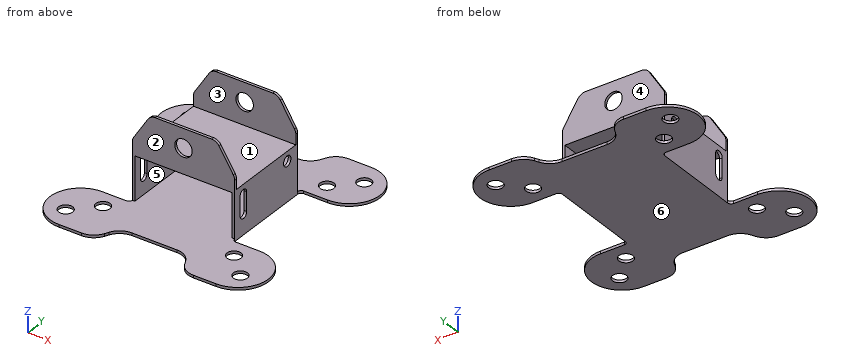
from build123d import *

# Parameters (mm, degrees)
SKETCH1_R           = 4.022928706
BOSS_EXTRUDE1_DEPTH = 1.5
SKETCH3_W           = 1.5
SKETCH3_H           = 50.876500294
BOSS_EXTRUDE2_DEPTH = 25
SKETCH4_W           = 58.54657641
SKETCH4_H           = 50.876500294
BOSS_EXTRUDE3_DEPTH = 1.5
SKETCH5_R           = 5
BOSS_EXTRUDE4_DEPTH = 1.5
SKETCH8_R           = 2.960999365
CUT_EXTRUDE1_DEPTH  = 92.835038059
FILLET1_R           = 5


with BuildPart() as part:
    # Sketch1 → Boss-Extrude1 (new body)
    with BuildSketch(Plane.XY):
        with BuildLine():
            Line((-31.273288205, 27.438250147), (-45, 27.438250147))
            ThreePointArc((-45, 27.438250147), (-62.561749853, 45), (-45, 62.561749853))
            Line((-45, 62.561749853), (-31.990503674, 62.561749853))
            ThreePointArc((-31.990503674, 62.561749853), (-26.633250489, 61.005673012), (-22.943256827, 56.821717516))
            Line((-22.943256827, 56.821717516), (-21.912531254, 54.632680079))
            ThreePointArc((-21.912531254, 54.632680079), (-18.222537592, 50.448724583), (-12.865284407, 48.892647742))
            Line((-12.865284407, 48.892647742), (12.865284407, 48.892647742))
            ThreePointArc((12.865284407, 48.892647742), (18.222537592, 50.448724583), (21.912531254, 54.632680079))
            Line((21.912531254, 54.632680079), (22.943256827, 56.821717516))
            ThreePointArc((22.943256827, 56.821717516), (26.633250489, 61.005673012), (31.990503674, 62.561749853))
            Line((31.990503674, 62.561749853), (45, 62.561749853))
            ThreePointArc((45, 62.561749853), (62.561749853, 45), (45, 27.438250147))
            Line((45, 27.438250147), (31.273288205, 27.438250147))
            ThreePointArc((31.273288205, 27.438250147), (29.859074643, 26.852463709), (29.273288205, 25.438250147))
            Line((29.273288205, 25.438250147), (29.273288205, -25.438250147))
            ThreePointArc((29.273288205, -25.438250147), (29.859074643, -26.852463709), (31.273288205, -27.438250147))
            Line((31.273288205, -27.438250147), (45, -27.438250147))
            ThreePointArc((45, -27.438250147), (62.561749853, -45), (45, -62.561749853))
            Line((45, -62.561749853), (31.990503674, -62.561749853))
            ThreePointArc((31.990503674, -62.561749853), (26.633250489, -61.005673012), (22.943256827, -56.821717516))
            Line((22.943256827, -56.821717516), (21.912531254, -54.632680079))
            ThreePointArc((21.912531254, -54.632680079), (18.222537592, -50.448724583), (12.865284407, -48.892647742))
            Line((12.865284407, -48.892647742), (-12.865284407, -48.892647742))
            ThreePointArc((-12.865284407, -48.892647742), (-18.222537592, -50.448724583), (-21.912531254, -54.632680079))
            Line((-21.912531254, -54.632680079), (-22.943256827, -56.821717516))
            ThreePointArc((-22.943256827, -56.821717516), (-26.633250489, -61.005673012), (-31.990503674, -62.561749853))
            Line((-31.990503674, -62.561749853), (-45, -62.561749853))
            ThreePointArc((-45, -62.561749853), (-62.561749853, -45), (-45, -27.438250147))
            Line((-45, -27.438250147), (-31.273288205, -27.438250147))
            ThreePointArc((-31.273288205, -27.438250147), (-29.859074643, -26.852463709), (-29.273288205, -25.438250147))
            Line((-29.273288205, -25.438250147), (-29.273288205, 25.438250147))
            ThreePointArc((-29.273288205, 25.438250147), (-29.859074643, 26.852463709), (-31.273288205, 27.438250147))
        make_face()
        with Locations((-50, 50)):
            Circle(SKETCH1_R, mode=Mode.SUBTRACT)
        with Locations((50, 50)):
            Circle(SKETCH1_R, mode=Mode.SUBTRACT)
        with Locations((-37.5, 37.5)):
            Circle(SKETCH1_R, mode=Mode.SUBTRACT)
        with Locations((37.5, 37.5)):
            Circle(SKETCH1_R, mode=Mode.SUBTRACT)
        with Locations((50, -50)):
            Circle(SKETCH1_R, mode=Mode.SUBTRACT)
        with Locations((37.5, -37.5)):
            Circle(SKETCH1_R, mode=Mode.SUBTRACT)
        with Locations((-37.5, -37.5)):
            Circle(SKETCH1_R, mode=Mode.SUBTRACT)
        with Locations((-50, -50)):
            Circle(SKETCH1_R, mode=Mode.SUBTRACT)
    extrude(amount=BOSS_EXTRUDE1_DEPTH)

    # Sketch3 → Boss-Extrude2 (add)
    with BuildSketch(Plane.XY.offset(1.5)):
        with Locations((-28.523288205, 0)):
            Rectangle(SKETCH3_W, SKETCH3_H)
        with Locations((28.523288205, 0)):
            Rectangle(SKETCH3_W, SKETCH3_H)
    extrude(amount=BOSS_EXTRUDE2_DEPTH)

    # Sketch4 → Boss-Extrude3 (add)
    with BuildSketch(Plane.XY.offset(26.5)):
        Rectangle(SKETCH4_W, SKETCH4_H)
    extrude(amount=BOSS_EXTRUDE3_DEPTH)

    # Sketch5 → Boss-Extrude4 (add)
    with BuildSketch(Plane(origin=(0, 25.438250147, 0), x_dir=(1, 0, 0), z_dir=(0, 1, 0))):
        Polygon((-29.273288205, -28), (-29.273288205, -35.308019153), (-18.871561113, -51.78577911), (18.871561113, -51.78577911), (29.273288205, -35.308019153), (29.273288205, -28), align=None)
        with Locations((0, -40.861297371)):
            Circle(SKETCH5_R, mode=Mode.SUBTRACT)
    boss_extrude4 = extrude(amount=-BOSS_EXTRUDE4_DEPTH)

    # Mirror1: Boss-Extrude4 across plane
    add(boss_extrude4.mirror(Plane.ZX))

    # Sketch8 → Cut-Extrude1 (cut, through all)
    with BuildSketch(Plane.ZY.offset(29.273288205)):
        with Locations((22.546846222, 17.00872447)):
            Circle(SKETCH8_R)
        with BuildLine():
            Line((11.727810079, -15.733095436), (22.546846222, -15.733095436))
            ThreePointArc((22.546846222, -15.733095436), (25.204153345, -18.390402559), (22.546846222, -21.047709682))
            Line((22.546846222, -21.047709682), (11.727810079, -21.047709682))
            ThreePointArc((11.727810079, -21.047709682), (9.070502956, -18.390402559), (11.727810079, -15.733095436))
        make_face()
    extrude(amount=-CUT_EXTRUDE1_DEPTH, mode=Mode.SUBTRACT)

    # Fillet1
    fillet1_edges = [part.edges().sort_by_distance(p)[0] for p in [
        (29.273288205, 24.688250147, 35.308019153),
        (18.871561113, 24.688250147, 51.78577911),
        (-18.871561113, 24.688250147, 51.78577911),
        (-29.273288205, 24.688250147, 35.308019153),
        (-29.273288205, -24.688250147, 35.308019153),
        (-18.871561113, -24.688250147, 51.78577911),
        (18.871561113, -24.688250147, 51.78577911),
        (29.273288205, -24.688250147, 35.308019153),
    ]]
    fillet(fillet1_edges, radius=FILLET1_R)


solid = part.part
Geometry: final body of the model. Coordinates: model frame, mm. Face numbers are marked on the shaded views. A direction names the side the tool comes from. Give positions to 0.01 mm unless a question says otherwise; leave off trailing zeros. Write each loop counter-clockwise with the first axis right and the second up, starting at its lowest first coordinate (ties: lowest second). Pieces come first, ordered by that corner, then holes. Notation, with made-up numbers: (74, 67) - (107, 67) arc R22 cw to (107, 73) - close; hole circle Ø4 at (8.25, 46.5). An arc over 180 degrees is marked (long way). Return JSON: item names as keys, results as strings. Group by question number.
1) Line query: line 1 (X direction, y = -20.5, z = 25.5); line 2 (Y direction, x = 16.5, z = 48.5); line 3 (Z direction, x = 0, y = -24.7). Output: solid intervals per line, ascending.
2) Section A-A on x = 0. Return the cut outline in (y, z).
3) Set-up query: the marked faces 5 and 6. Return all of +Z, -Z, +X, -X, +Y, -Y with unobstructed straight access to the full face (end or side cutting, diameter ignored); none if empty.
4) Mould query, pull axis Y, two halves, no side actions, for the marked faces 1, 2, 3 and 4. Classes: released by +Y, released by -Y, zero draft, split by the parting line, or undercut.
5) Section C-C on x = -43. Return the cut outline in (y, z), plus the area to 3 significant figures.
6) Section D-D on y = -0.5. Return the cut outline in (x, z), plus the area to 3 significant figures.
7) First-contact query: P1, Ø12, axis at y = 19, z = 18, coming from the -X side; P2, Ø3, axis at x = 32, y = -8.5, coming from the +Z side; P3, Ø5, axis at y = -8.5, z = 8.5, coming from the +X side; P4, Ø2, axis at x = 28, y = -32, coming from the +Z side. Flat tips, straight axial feed; report the tip coordinate or a pass-through.
8) Section B-B on z = 3. Return the cut outline in (x, y).
Filled in:
{
 "1": {"line 1": "x = -29.27 to -27.77, 27.77 to 29.27", "line 2": "y = -25.44 to -23.94, 23.94 to 25.44", "line 3": "z = 0 to 1.5, 26.5 to 35.86, 45.86 to 51.79"},
 "2": {"outline": "(-48.89, 0) - (48.89, 0) - (48.89, 1.5) - (-48.89, 1.5) - close; (-25.44, 26.5) - (25.44, 26.5) - (25.44, 35.86) - (23.94, 35.86) - (23.94, 28) - (-23.94, 28) - (-23.94, 35.86) - (-25.44, 35.86) - close; (-25.44, 45.86) - (-23.94, 45.86) - (-23.94, 51.79) - (-25.44, 51.79) - close; (23.94, 45.86) - (25.44, 45.86) - (25.44, 51.79) - (23.94, 51.79) - close"},
 "3": {"face 5": "+Y, -Y", "face 6": "-Z, +X, -X, +Y, -Y"},
 "4": {"face 1": "undercut", "face 2": "released by -Y", "face 3": "undercut", "face 4": "released by +Y"},
 "5": {"outline": "(-62.56, 0) - (-27.44, 0) - (-27.44, 1.5) - (-62.56, 1.5) - close; (27.44, 0) - (62.56, 0) - (62.56, 1.5) - (27.44, 1.5) - close", "area": "105 mm^2"},
 "6": {"outline": "(-29.27, 0) - (29.27, 0) - (29.27, 28) - (-29.27, 28) - close; hole (-27.77, 1.5) - (27.77, 1.5) - (27.77, 26.5) - (-27.77, 26.5) - close", "area": "251 mm^2"},
 "7": {"P1": "stops at x = -29.27", "P2": "passes through", "P3": "stops at x = 29.27", "P4": "stops at z = 1.5"},
 "8": {"outline": "(-29.27, -25.44) - (-27.77, -25.44) - (-27.77, 25.44) - (-29.27, 25.44) - close; (27.77, -25.44) - (29.27, -25.44) - (29.27, 25.44) - (27.77, 25.44) - close"}
}
